Read the model definition and answer for the solid it produces. Units are mm, in the model's axes. A direction names the side the tool comes from. Round coordinates to 2 decimals unless told otherwise and drop trailing zeros. Order: outer loops, then holes, each group sorted by start corner. A loop starts at its lowest first (then second) coordinate and runs counter-clockwise, first axis right, second up. Notation, with made-up numbers: M 5,2.5 L 33,2.5 A17 cw 33,34.5 Z; hole C -31,-21 d5. An arc over 180 degrees is marked long. Use one line per item in the form item = value. Start each with the question number.
from build123d import *


with BuildPart() as part:
    # Esquisse1 → Base-Révolution (revolve)
    with BuildSketch(Plane.XY, mode=Mode.PRIVATE) as base_r_volution_sk:
        Polygon((0, 7.334147334), (0, 9.634147334), (11, 9.634147334), (11, 7.334147334), (8.8, 7.334147334), (8.8, 5.134147334), (2.2, 5.134147334), (2.2, 7.334147334), align=None)
    revolve(base_r_volution_sk.sketch.rotate(Axis((-12.574722565, 0.134147334, 0), (1, 0, 0)), 90), axis=Axis((-12.574722565, 0.134147334, 0), (1, 0, 0)))


solid = part.part
Item 1: Section D-D (y = 8.5) is taken. Write down the section's boundary in (x, z).
Item 2: Section A-A (z = 0) is taken. Write down the section's boundary in (x, y).
Item 3: Given P1, Ø9, axis at y = 0.13, z = 0, coming from the -X side; P2, Ø3, axis at x = 8.5, y = -5, coming from the -Z side; P3, Ø5, axis at x = 8, z = -3, coming from the +Y side; P4, Ø5, axis at y = 2.5, z = -4, coming from the -X side, each flat-ended and moving along its own axis, determine where each tip first touches the part or whether it passes through.
Item 4: A tool of negligible diameter and unlimited length cuts with its end or side. For faces 1 (the cylindrical face through (1.085, -2.029, 6.868)), 2 (the flat face through (8.8, 2, -5)), 3 (the cylindrical face through (5.454, -4.823, -0.651)), from which of +Z, -Z, +X, -X, +Y, -Y can it reach the whole face along a straight path? Write none if from no direction.
Item 5: For a pull along Y with two mould halves and no side action, classify faces 4 (the cylindrical face through (5.58, -2.72, 9.06)), 5 (the cylindrical face through (9.885, -2.029, 6.868)), 6 (the flat face through (11, -2, -7.1)) as pulls with the +Y half, pulls with the -Y half, needs draft (parallel to the pull), parting line crosses it, or undercut.
Item 6: Find the intervals of material crossed by L1, parallel to Z at x = 2.25, y = 0; L2, parallel to Y at x = 10.1, z = 0; L3, parallel to X at y = -5.25, z = 2, in increasing order. Write a range as [from, to].
Item 7: Section C-C (z = 2.5) is taken. Write down the section's boundary in (x, y).
Item 8: Section B-B (x = 7.5) is taken. Write down the section's boundary in (y, z).
The answers:
q1.outline = M 0,-4.5 L 11,-4.5 L 11,4.5 L 0,4.5 Z
q2.outline = M 0,-9.37 L 11,-9.37 L 11,-7.07 L 8.8,-7.07 L 8.8,-4.87 L 2.2,-4.87 L 2.2,-7.07 L 0,-7.07 Z; M 0,7.33 L 2.2,7.33 L 2.2,5.13 L 8.8,5.13 L 8.8,7.33 L 11,7.33 L 11,9.63 L 0,9.63 Z
q3.P1 = through
q3.P2 = -8.78
q3.P3 = 9.62
q3.P4 = 2.2
q4.face_1 = -X
q4.face_2 = +X
q4.face_3 = +X, -X
q5.face_4 = parting line crosses it
q5.face_5 = undercut
q5.face_6 = needs draft
q6.L1 = [-9.5, -5], [5, 9.5]
q6.L2 = [-9.37, -7.07], [7.33, 9.63]
q6.L3 = [2.2, 8.8]
q7.outline = M 0,-9.03 L 11,-9.03 L 11,-6.62 L 8.8,-6.62 L 8.8,-4.2 L 2.2,-4.2 L 2.2,-6.62 L 0,-6.62 Z; M 0,6.89 L 2.2,6.89 L 2.2,4.46 L 8.8,4.46 L 8.8,6.89 L 11,6.89 L 11,9.3 L 0,9.3 Z
q8.outline = C 0.13,0 d19; hole C 0.13,0 d10
